Design review of the part shown in the three views and the two pictorial views. Dimensions are in mm from the part's minimum x, y and z. Give positions to 0.01 mm unless a question says otherwise; leave off trailing zeros. Order: outer loops, then holes, each group sorted by start corner. A loop starts at its lowest first (then second) coordinate and runs counter-clockwise, first axis right, second up. Notation, with made-up numbers: (20, 34.25) -> (56, 34.25) arc R14 ccw to (56, 46.25) -> close; hole circle Ø1 at (16, 60.25). An arc over 180 degrees is marked (long way). Use one line per item in the form item = value.
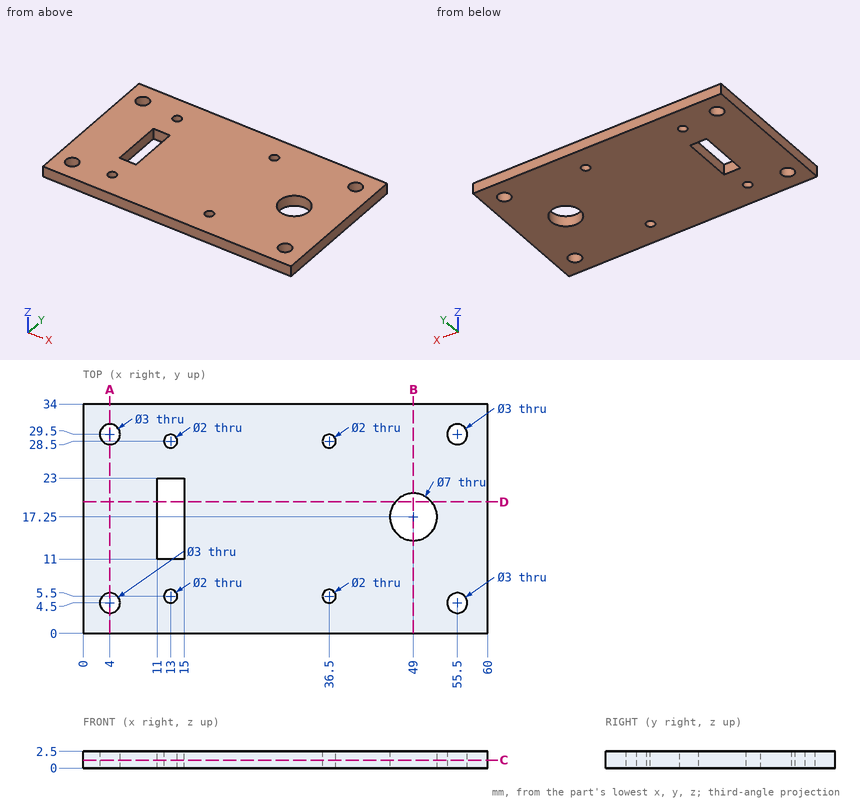
1. Add section B-B on x = 49. Give the boundary of the cut face in (y, z), then the cut area to 3 significant figures.
Values:
outline = (0, 0) -> (13.75, 0) -> (13.75, 2.5) -> (0, 2.5) -> close; (20.75, 0) -> (34, 0) -> (34, 2.5) -> (20.75, 2.5) -> close
area = 67.5 mm^2
2. For pin 1 Ø1.2 at (x, y) = (13, 5.5) entering from -Z, flat-tipped, find the tip position at first contact; note if it passes through.
Values:
pin_1 = through
3. Add section C-C on z = 1.2. Count the separate pieces of the cut face and the enclosed holes in it, then the cut area to 3 significant figures.
Values:
separate_pieces = 1
enclosed_holes = 10
area = 1,910 mm^2
4. Add section A-A on x = 4. Give the boundary of the cut face in (y, z), then the cut area to 3 significant figures.
Values:
outline = (0, 0) -> (3, 0) -> (3, 2.5) -> (0, 2.5) -> close; (6, 0) -> (28, 0) -> (28, 2.5) -> (6, 2.5) -> close; (31, 0) -> (34, 0) -> (34, 2.5) -> (31, 2.5) -> close
area = 70.0 mm^2
5. Add section D-D on y = 19.5. Give the boundary of the cut face in (x, z).
Values:
outline = (0, 0) -> (11, 0) -> (11, 2.5) -> (0, 2.5) -> close; (15, 0) -> (46.32, 0) -> (46.32, 2.5) -> (15, 2.5) -> close; (51.68, 0) -> (60, 0) -> (60, 2.5) -> (51.68, 2.5) -> close
6. For L1, parallel to Y at x = 13, z = 1.6; L2, parallel to X at y = 17, z = 0.75; L3, parallel to X at y = 22.5, z = 1.4, list the stretches that pass through material, from the lowest coordinate up.
Values:
L1 = 0 to 4.5, 6.5 to 11, 23 to 27.5, 29.5 to 34
L2 = 0 to 11, 15 to 45.51, 52.49 to 60
L3 = 0 to 11, 15 to 60
